The listing builds one solid part. Answer for the finished solid, in the listing's coordinates (mm). A direction names the side the tool comes from. Coordinates: 2 decimals unless noted, no trailing zeros. Loops run counter-clockwise (first coordinate to the right, second up) from the corner with the lowest first, then second, coordinate; pieces in that order, holes last. Notation, with made-up numbers: M -7,9.5 L 17,9.5 A17 cw 17,18.5 Z; hole C -14,-7 d4. An arc over 180 degrees is marked long. Answer as a JSON object with one key per item and string values. Group by question number.
1. Determine the mould class of faces 4 (the face through (0.24, -14.45, 3.13)), 5 (the face through (-0.5, 2.23, 3.13)), 6 (the face through (14.88, 11.85, 1.37)) for opening direction X: released by +X, released by -X, zero draft, split by the parting line, or undercut.
2. A cutting plane is placed at D-D on x = -1.5. Give the vertices of the cut face in (y, z).
3. A cutting plane is placed at B-B on y = -5. Give the vertices of the cut face in (x, z).
4. Straight lines are drawn through the part: L1, parallel to Y at x = 11.43, z = 3.8 (3 decimals); L2, parallel to Z at x = 6, y = 4.5; L3, parallel to Y at x = 0, z = 2. For each, find the intervals that lie inside material, in ascending order.
5. A cutting plane is placed at C-C on z = 3.25. Give the vertices of the cut face in (x, y) (3 decimals).
6. Given pin 1 (4 mm diameter, centred on y = -8, z = -2.5, fed in from -X); pin 2 (2.5 mm diameter, centred on x = 10, y = -7.5, fed in from -Z); pin 3 (1.5 mm diameter, centred on x = -1, y = -5.5, fed in from -Z), each flat-ended and moving along its own axis, determine where each tip first touches the part or whether it passes through.
7. For faces 1 (the face through (13.2, -8.1, 2.54)), 2 (the face through (9.146, -6.451, 4.418)), 3 (the face through (14.986, 4, -3)), determine the directions among +Z, -Z, +X, -X, +Y, -Y from which every point of the face is accessible in a straight line to the end or side of a thin tool.
Autodesk Inventor part; units mm, degrees
ref_plane "YZ Plane" through (0, 0, 0) normal (1, 0, 0) x (0, 1, 0)
ref_plane "XZ Plane" through (0, 0, 0) normal (0, 1, 0) x (-1, 0, 0)
ref_plane "XY Plane" through (0, 0, 0) normal (0, 0, 1) x (1, 0, 0)
sketch "Sketch1" plane through (0, 0, 0) normal (0, 0, 1) x (1, 0, 0)
  line L0 (12.7, -12.7) -> (-12.7, -12.7)
  line L1 (-12.7, -12.7) -> (-12.7, 12.7)
  line L2 (-12.7, 12.7) -> (12.7, 12.7)
  line L3 (12.7, 12.7) -> (12.7, -12.7)
  line L4 (12.7, -12.7) -> (-12.7, 12.7) construction
  line L5 (-12.7, -12.7) -> (12.7, 12.7) construction
  circle A0 centre (11.43, -6.35) radius 9.525
  line L6 (12.7, 12.7) -> (14.986, 12.7)
  line L7 (14.986, 12.7) -> (14.986, -15.1863)
  line L8 (14.986, -12.7) -> (12.7, -12.7)
  line L9 (12.7, -12.7) -> (12.7, 12.7) construction
  line L10 (6.6364, -7.4249) -> (8.1023, -2.736) construction
  line L11 (8.1023, -2.736) -> (12.8959, -1.6611) construction
  line L12 (12.8959, -1.6611) -> (16.2236, -5.2751) construction
  line L13 (16.2236, -5.2751) -> (14.7577, -9.964) construction
  line L14 (14.7577, -9.964) -> (9.9641, -11.0389) construction
  line L15 (9.9641, -11.0389) -> (6.6364, -7.4249) construction
  circle A1 centre (11.43, -6.35) radius 2.286
  circle A2 centre (11.43, -6.35) radius 4.0005
  circle A3 centre (0, 0) radius 2.286
  line L16 (10.1541, -15.7892) -> (-12.7, -12.7)
  line L17 (14.986, 12.7) -> (20.4433, -3.27)
  point P0 (14.986, -9.2337)
  point P1 (14.986, -4.5173)
  point P2 (14.986, -8.1827)
  point P3 (12.1553, 12.7)
  point P4 (-5.8053, 12.7)
  point P5 (4.3305, -12.7)
  point P6 (12.7, 3.09)
  point P7 (14.986, 2.4863)
  dimension "d0" = 25.4
  dimension "d1" = 25.4
  dimension "d3" = 19.05
  dimension "d5" = 8.509
  dimension "d6" = 4.572
  dimension "d13" = 8.001
  dimension "d17" = 4.572
  dimension "d19" = 2.286
  dimension "d26" = 6.35
  dimension "d27" = 11.43
extrude "Extrusion1" add sketch "Sketch1" along normal blind 6.35 contours L8 L7 A0 L0 | L0 A0 L3 A2 | L3 A2 L7 L8 | A0 L16 L0 | L0 L1 L2 L3 A0 | A2 L3 A1 | L3 A1 A2 L7 | L7 A2 A0 | A0 L7 A2 L3 | L3 L6 L7 A0 | L7 A2 | L7 L17 A0
extrude "Extrusion2" add sketch "Sketch1" against normal blind 6.35 contours L7 A2 A0 | L7 L17 A0
extrude "Extrusion3" cut sketch "Sketch1" along normal blind 2.54 contours A2 L3 A1 | L3 A1 A2 L7 | L7 A2
fillet "Fillet2" radius 3.175 3 edges at (14.986, 12.7, 3.175) (-12.7, -12.7, 3.175) (-12.7, 12.7, 3.175)
fillet "Fillet1" radius 1.27 1 edges at (14.986, 3.6136, -6.35)
properties part number "Elevator Tensioner"
From the geometry:
{
 "1": {"face 4": "released by -X", "face 5": "undercut", "face 6": "released by +X"},
 "2": {"outline": "M -14.21,0 L -1.73,0 L -1.73,6.35 L -14.21,6.35 Z; M 1.73,0 L 12.7,0 L 12.7,6.35 L 1.73,6.35 Z"},
 "3": {"outline": "M -12.7,0 L 7.66,0 L 7.66,2.54 L 9.59,2.54 L 9.59,6.35 L -12.7,6.35 Z; M 13.27,2.54 L 15.2,2.54 L 15.2,-5.78 A1.27 ccw 16.26,-6.35 L 20.86,-6.35 L 20.86,6.35 L 13.27,6.35 Z"},
 "4": {"L1": "y = -15.875 to -8.636, -4.064 to 12.7", "L2": "z = 0 to 6.35", "L3": "y = -14.42 to -2.29, 2.29 to 12.7"},
 "5": {"outline": "M -12.7,-9.925 A3.175 ccw -9.95,-13.072 L 10.154,-15.789 A9.525 ccw 20.443,-3.27 L 15.72,10.552 A3.175 ccw 12.716,12.7 L -9.525,12.7 A3.175 ccw -12.7,9.525 Z; hole C 0,0 d4.572; hole C 11.43,-6.35 d4.572"},
 "6": {"pin 1": "stops at x = 14.99", "pin 2": "stops at z = 2.54", "pin 3": "stops at z = 0"},
 "7": {"face 1": "-Z", "face 2": "+Z, -Z", "face 3": "-Z, -X, +Y, -Y"}
}
